from build123d import *

# Parameters (mm, degrees)
SKETCH_1_R          = 5
SKETCH_1_R_2        = 3
EXTRUDE_1_DEPTH     = 21.8
SKETCH_2_W          = 16
SKETCH_2_H          = 7
EXTRUDE_2_DEPTH     = 21.8
SKETCH_3_W          = 12
SKETCH_3_H          = 3
CUT_EXTRUDE_1_DEPTH = 22
SKETCH_4_R          = 1.65
CUT_EXTRUDE_2_DEPTH = 22


with BuildPart() as part:
    # 草图1 → 凸台-拉伸1 (new body)
    with BuildSketch(Plane(origin=(0, 0, 0), x_dir=(1, 0, 0), z_dir=(0, 1, 0))):
        with Locations(Location((0, 0, 0), (0, 0, 270))):
            Circle(SKETCH_1_R)
        with Locations(Location((0, 0, 0), (0, 0, 270))):
            Circle(SKETCH_1_R_2, mode=Mode.SUBTRACT)
    extrude(amount=EXTRUDE_1_DEPTH)

    # 草图2 → 凸台-拉伸2 (add)
    with BuildSketch(Plane(origin=(0, 21.8, 0), x_dir=(1, 0, 0), z_dir=(0, 1, 0))):
        with Locations((11.1, 0)):
            Rectangle(SKETCH_2_W, SKETCH_2_H)
    extrude(amount=-EXTRUDE_2_DEPTH)

    # 草图3 → 切除-拉伸1 (cut)
    with BuildSketch(Plane(origin=(0, 21.8, 0), x_dir=(1, 0, 0), z_dir=(0, 1, 0))):
        with Locations((13.1, 0)):
            Rectangle(SKETCH_3_W, SKETCH_3_H)
    extrude(amount=-CUT_EXTRUDE_1_DEPTH, mode=Mode.SUBTRACT)

    # 草图4 → 切除-拉伸2 (cut)
    with BuildSketch(Plane.XY.offset(3.5)):
        with Locations(Location((13.1, 14.9, 0), (0, 0, 180))):
            Circle(SKETCH_4_R)
        with Locations(Location((13.1, 6.9, 0), (0, 0, 180))):
            Circle(SKETCH_4_R)
    extrude(amount=-CUT_EXTRUDE_2_DEPTH, mode=Mode.SUBTRACT)


solid = part.part
Here's how the part is built. I have some questions about the finished solid (model axes, mm). A direction names the side the tool comes from. Give positions to 0.01 mm unless a question says otherwise; leave off trailing zeros. Order: outer loops, then holes, each group sorted by start corner. A loop starts at its lowest first (then second) coordinate and runs counter-clockwise, first axis right, second up. Notation, with made-up numbers: M 37.5,0.25 L 84.5,0.25 A27 ccw 84.5,37.25 Z; hole C 53,20 d11. An arc over 180 degrees is marked long. Answer as a JSON object with one key per item and string values. Group by question number.
1) Suppose I cut it at C-C, the plane x = 0. Write out the boundary of the cut face in (y, z), plus the area to 3 significant figures.
2) Suppose I cut it at B-B, the plane z = 0. Write out the boundary of the cut face in (x, y), plus the area to 3 significant figures.
3) We'd pull the mould along X, two halves only. Please class faces 4 (the flat face through (11, 11, -3.5)), 5 (the flat face through (19.1, 11, -2)), 6 (the cylindrical face through (14.75, 6.83, -2.49)), 7 (the cylindrical face through (0.9, 10.75, 2.86)): pulls with the +X half, pulls with the -X half, needs draft (parallel to the pull), parting line crosses it, or undercut.
4) Suppose I cut it at D-D, the plane y = 11. Write out the boundary of the cut face in (x, z).
5) Please list where these lines run through material, in increasing order: L1, parallel to Y at x = 13.1, z = -2.2; L2, parallel to Z at x = 9, y = 5.75; L3, parallel to Z at x = 5, y = 12.25. Write a range as [from, to].
6) I'm going to push flat-ended pins straight in: pin 1 Ø8 at (x, y) = (8, 8) entering from -Z; pin 2 Ø3 at (x, y) = (13.1, 6.9) entering from -Z; pin 3 Ø13 at (x, y) = (11, 14) entering from +Z; pin 4 Ø1 at (y, z) = (8, -0.5) entering from +X. Where does each tip first touch, or does it pass through?
7) On a 3-axis mill with a long thin cutter (end or side, diameter ignored), from which of +Z, -Z, +X, -X, +Y, -Y can I reach the whole of each face in a straight line? I mean faces 1 (the flat face through (5, 0, 0)), 2 (the flat face through (11, 11, 3.5)), 3 (the flat face through (13, 11, 1.5)). Say none if no direction works.
8) Suppose I cut it at A-A, the plane y = 6.9. Write out the boundary of the cut face in (x, z), plus the area to 3 significant figures.
Results found:
{
 "1": {"outline": "M 0,-5 L 21.8,-5 L 21.8,-3 L 0,-3 Z; M 0,3 L 21.8,3 L 21.8,5 L 0,5 Z", "area": "87.2 mm²"},
 "2": {"outline": "M -5,0 L -3,0 L -3,21.8 L -5,21.8 Z; M 3,0 L 7.1,0 L 7.1,21.8 L 3,21.8 Z", "area": "133 mm²"},
 "3": {"face 4": "needs draft", "face 5": "pulls with the +X half", "face 6": "undercut", "face 7": "undercut"},
 "4": {"outline": "M 3.57,-3.5 L 19.1,-3.5 L 19.1,-1.5 L 7.1,-1.5 L 7.1,1.5 L 19.1,1.5 L 19.1,3.5 L 3.57,3.5 A5 ccw long Z; hole C 0,0 d6"},
 "5": {"L1": "[0, 5.25], [8.55, 13.25], [16.55, 21.8]", "L2": "[-3.5, -1.5], [1.5, 3.5]", "L3": "[-3.5, 3.5]"},
 "6": {"pin 1": "z = -3.5", "pin 2": "through", "pin 3": "z = 3.5", "pin 4": "x = 7.1"},
 "7": {"face 1": "+Z, -Z, +X, -X, -Y", "face 2": "+Z, +X, +Y, -Y", "face 3": "+X, +Y, -Y"},
 "8": {"outline": "M 3.57,-3.5 L 11.45,-3.5 L 11.45,-1.5 L 7.1,-1.5 L 7.1,1.5 L 11.45,1.5 L 11.45,3.5 L 3.57,3.5 A5 ccw long Z; M 14.75,-3.5 L 19.1,-3.5 L 19.1,-1.5 L 14.75,-1.5 Z; M 14.75,1.5 L 19.1,1.5 L 19.1,3.5 L 14.75,3.5 Z; hole C 0,0 d6", "area": "103 mm²"}
}
